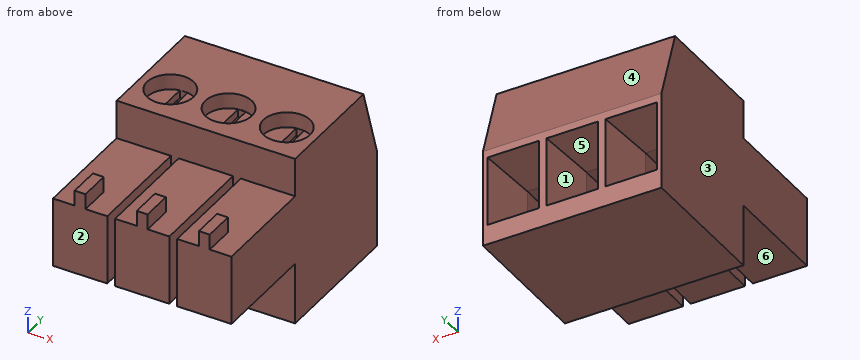
from build123d import *

# Parameters (mm, degrees)
SKETCH1_W                    = 11.5
SKETCH1_H                    = 11
BOSS_EXTRUDE1_DEPTH          = 9
SKETCH2_W                    = 3.5
SKETCH2_H                    = 4.5
BOSS_EXTRUDE2_DEPTH          = 7
SKETCH3_W                    = 3.3
SKETCH3_H                    = 4.5
CUT_EXTRUDE1_DEPTH           = 3
CUT_EXTRUDE1_DRAFT           = -15
CUT_EXTRUDE1_PROFILE_2_DEPTH = 3
CUT_EXTRUDE1_PROFILE_2_DRAFT = -15
CUT_EXTRUDE1_PROFILE_3_DEPTH = 3
CUT_EXTRUDE1_PROFILE_3_DRAFT = -15
SKETCH4_W                    = 1.692304846
SKETCH4_H                    = 2.892304846
CUT_EXTRUDE2_DEPTH           = 3
CUT_EXTRUDE3_DEPTH           = 17
SKETCH6_R                    = 1.5
CUT_EXTRUDE4_DEPTH           = 1
SKETCH7_W                    = 0.5
SKETCH7_H                    = 2.958039891
CUT_EXTRUDE5_DEPTH           = 0.5
SKETCH8_W                    = 0.7
SKETCH8_H                    = 2
BOSS_EXTRUDE3_DEPTH          = 1


with BuildPart() as part:
    # Sketch1 → Boss-Extrude1 (new body)
    with BuildSketch(Plane(origin=(0, 0, 0), x_dir=(1, 0, 0), z_dir=(0, 1, 0))):
        Rectangle(SKETCH1_W, SKETCH1_H)
    extrude(amount=BOSS_EXTRUDE1_DEPTH)

    # Sketch2 → Boss-Extrude2 (add)
    with BuildSketch(Plane.XZ):
        with Locations((-4, 0.75)):
            Rectangle(SKETCH2_W, SKETCH2_H)
        with Locations((4, 0.75)):
            Rectangle(SKETCH2_W, SKETCH2_H)
        with Locations((0, 0.75)):
            Rectangle(SKETCH2_W, SKETCH2_H)
    extrude(amount=BOSS_EXTRUDE2_DEPTH)


with BuildPart() as cut_extrude1_tool:
    # Sketch3 → Cut-Extrude1 (with draft: the straight prism first)
    with BuildSketch(Plane(origin=(0, 9, 0), x_dir=(1, 0, 0), z_dir=(0, 1, 0))):
        with Locations((3.8, 1.95)):
            Rectangle(SKETCH3_W, SKETCH3_H)
    extrude(amount=-CUT_EXTRUDE1_DEPTH)
    # Cut-Extrude1: the draft: its side faces are tilted about the plane it starts from
    cut_extrude1_sides = [cut_extrude1_tool.faces().sort_by_distance(p)[0] for p in [
        (3.8, 7.5, -4.2),
        (2.15, 7.5, -1.95),
        (3.8, 7.5, 0.3),
        (5.45, 7.5, -1.95),
    ]]
    draft(cut_extrude1_sides, Plane(origin=(0, 9, 0), x_dir=(1, 0, 0), z_dir=(0, 1, 0)), CUT_EXTRUDE1_DRAFT)


with BuildPart() as part_1:
    add(part.part)

    # Cut-Extrude1: cut by cut_extrude1_tool
    add(cut_extrude1_tool.part, mode=Mode.SUBTRACT)


with BuildPart() as cut_extrude1_profile_2_tool:
    # Sketch3 → Cut-Extrude1 profile 2 (with draft: the straight prism first)
    with BuildSketch(Plane(origin=(0, 9, 0), x_dir=(1, 0, 0), z_dir=(0, 1, 0))):
        with Locations((-3.8, 1.95)):
            Rectangle(SKETCH3_W, SKETCH3_H)
    extrude(amount=-CUT_EXTRUDE1_PROFILE_2_DEPTH)
    # Cut-Extrude1 profile 2: the draft: its side faces are tilted about the plane it starts from
    cut_extrude1_profile_2_sides = [cut_extrude1_profile_2_tool.faces().sort_by_distance(p)[0] for p in [
        (-3.8, 7.5, -4.2),
        (-5.45, 7.5, -1.95),
        (-3.8, 7.5, 0.3),
        (-2.15, 7.5, -1.95),
    ]]
    draft(cut_extrude1_profile_2_sides, Plane(origin=(0, 9, 0), x_dir=(1, 0, 0), z_dir=(0, 1, 0)), CUT_EXTRUDE1_PROFILE_2_DRAFT)


with BuildPart() as part_2:
    add(part_1.part)

    # Cut-Extrude1 profile 2: cut by cut_extrude1_profile_2_tool
    add(cut_extrude1_profile_2_tool.part, mode=Mode.SUBTRACT)


with BuildPart() as cut_extrude1_profile_3_tool:
    # Sketch3 → Cut-Extrude1 profile 3 (with draft: the straight prism first)
    with BuildSketch(Plane(origin=(0, 9, 0), x_dir=(1, 0, 0), z_dir=(0, 1, 0))):
        with Locations((0, 1.95)):
            Rectangle(SKETCH3_W, SKETCH3_H)
    extrude(amount=-CUT_EXTRUDE1_PROFILE_3_DEPTH)
    # Cut-Extrude1 profile 3: the draft: its side faces are tilted about the plane it starts from
    cut_extrude1_profile_3_sides = [cut_extrude1_profile_3_tool.faces().sort_by_distance(p)[0] for p in [
        (-1.65, 7.5, -1.95),
        (0, 7.5, 0.3),
        (1.65, 7.5, -1.95),
        (0, 7.5, -4.2),
    ]]
    draft(cut_extrude1_profile_3_sides, Plane(origin=(0, 9, 0), x_dir=(1, 0, 0), z_dir=(0, 1, 0)), CUT_EXTRUDE1_PROFILE_3_DRAFT)


with BuildPart() as part_3:
    add(part_2.part)

    # Cut-Extrude1 profile 3: cut by cut_extrude1_profile_3_tool
    add(cut_extrude1_profile_3_tool.part, mode=Mode.SUBTRACT)

    # Sketch4 → Cut-Extrude2 (cut)
    with BuildSketch(Plane(origin=(0, 6, 0), x_dir=(1, 0, 0), z_dir=(0, 1, 0))):
        with Locations((-3.8, 1.95)):
            Rectangle(SKETCH4_W, SKETCH4_H)
        with Locations((3.8, 1.95)):
            Rectangle(SKETCH4_W, SKETCH4_H)
        with Locations((0, 1.95)):
            Rectangle(SKETCH4_W, SKETCH4_H)
    extrude(amount=-CUT_EXTRUDE2_DEPTH, mode=Mode.SUBTRACT)

    # Sketch5 → Cut-Extrude3 (cut)
    with BuildSketch(Plane.ZY.offset(5.75)):
        Polygon((5.5, 9), (0.8, 9), (5.5, 7.5), align=None)
    extrude(amount=-CUT_EXTRUDE3_DEPTH, mode=Mode.SUBTRACT)

    # Sketch6 → Cut-Extrude4 (cut)
    with BuildSketch(Plane.XY.offset(5.5)):
        with Locations((-3.75, 2.487199689)):
            Circle(SKETCH6_R)
        with Locations((0, 2.487199689)):
            Circle(SKETCH6_R)
        with Locations((3.75, 2.487199689)):
            Circle(SKETCH6_R)
    extrude(amount=-CUT_EXTRUDE4_DEPTH, mode=Mode.SUBTRACT)

    # Sketch7 → Cut-Extrude5 (cut)
    with BuildSketch(Plane.XY.offset(4.5)):
        with Locations((-3.75, 2.487199689)):
            Rectangle(SKETCH7_W, SKETCH7_H)
        with Locations((0, 2.487199689)):
            Rectangle(SKETCH7_W, SKETCH7_H)
        with Locations((3.75, 2.487199689)):
            Rectangle(SKETCH7_W, SKETCH7_H)
    extrude(amount=-CUT_EXTRUDE5_DEPTH, mode=Mode.SUBTRACT)

    # Sketch8 → Boss-Extrude3 (add)
    with BuildSketch(Plane.XY.offset(3)):
        with Locations((4, -6)):
            Rectangle(SKETCH8_W, SKETCH8_H)
        with Locations((-4, -6)):
            Rectangle(SKETCH8_W, SKETCH8_H)
        with Locations((0, -6)):
            Rectangle(SKETCH8_W, SKETCH8_H)
    extrude(amount=BOSS_EXTRUDE3_DEPTH)


solid = part_3.part
Geometry: final body of the model. Coordinates: model frame, mm. Face numbers are marked on the shaded views. A direction names the side the tool comes from. Give positions to 0.01 mm unless a question says otherwise; leave off trailing zeros. Order: outer loops, then holes, each group sorted by start corner. A loop starts at its lowest first (then second) coordinate and runs counter-clockwise, first axis right, second up. Notation, with made-up numbers: (31.25, 71) -> (49.25, 71) arc R19 ccw to (49.25, 94) -> close; hole circle Ø10 at (44.25, 14). An arc over 180 degrees is marked (long way). Answer as a JSON object with one key per item and string values.
Q1. Material intervals for probe 1 along X at (y, z) = (-0.25, -0.25); probe 2 along Z at (x, y) = (-4, 4); probe 3 along X at (y, z) = (7, -1.25), sorted ascending.
Entries:
{"probe 1": "x = -5.75 to -2.25, -1.75 to 1.75, 2.25 to 5.75", "probe 2": "z = -5.5 to -3.4, -0.5 to 5.5", "probe 3": "x = -5.75 to -4.91, -2.69 to -1.11, 1.11 to 2.69, 4.91 to 5.75"}
Q2. Section A-A (y = 5.5). Output: boundary loops of the cut face in (x, z).
Entries:
{"outline": "(-5.75, -5.5) -> (5.75, -5.5) -> (5.75, 5.5) -> (-5.75, 5.5) -> close; hole (-4.65, -3.4) -> (-2.95, -3.4) -> (-2.95, -0.5) -> (-4.65, -0.5) -> close; hole (-0.85, -3.4) -> (0.85, -3.4) -> (0.85, -0.5) -> (-0.85, -0.5) -> close; hole (2.95, -3.4) -> (4.65, -3.4) -> (4.65, -0.5) -> (2.95, -0.5) -> close"}
Q3. Draft query along X for the marked faces 1, 2 and 3. Return one class per face: released by +X, released by -X, zero draft, split by the parting line, or undercut.
Entries:
{"face 1": "undercut", "face 2": "zero draft", "face 3": "released by -X"}
Q4. Section D-D (z = 1.75). Output: boundary loops of the cut face in (x, y), plus the area to 3 significant figures.
Entries:
{"outline": "(-5.75, -7) -> (-2.25, -7) -> (-2.25, 0) -> (-1.75, 0) -> (-1.75, -7) -> (1.75, -7) -> (1.75, 0) -> (2.25, 0) -> (2.25, -7) -> (5.75, -7) -> (5.75, 8.7) -> (-5.75, 8.7) -> close", "area": "174 mm^2"}
Q5. Access query for the marked faces 4, 5 and 6. Directions: +Z, -Z, +X, -X, +Y, -Y. A direction counts if a zero-diameter tool reaches every point of the face in a straight line with its end or side. Return the directions, or none.
Entries:
{"face 4": "+Z, +X, -X, +Y", "face 5": "+Y", "face 6": "-Z, +X, -X, -Y"}
Q6. Section B-B (y = -1). Output: boundary loops of the cut face in (x, z), plus the area to 4 significant figures.
Entries:
{"outline": "(-5.75, -1.5) -> (-2.25, -1.5) -> (-2.25, 3) -> (-5.75, 3) -> close; (-1.75, -1.5) -> (1.75, -1.5) -> (1.75, 3) -> (-1.75, 3) -> close; (2.25, -1.5) -> (5.75, -1.5) -> (5.75, 3) -> (2.25, 3) -> close", "area": "47.25 mm^2"}
Q7. First-contact query: pin 1 (0.6 mm diameter, centred on x = 4, z = 4.5, fed in from -Y); pin 2 (1 mm diameter, centred on x = -4.5, y = -3, fed in from +Z); pin 3 (2 mm diameter, centred on x = -0.5, z = 1, fed in from +Y); pin 4 (4 mm diameter, centred on x = 4, y = -4.5, fed in from +Z). Flat tips, straight axial feed; report the tip coordinate or a pass-through.
Entries:
{"pin 1": "stops at y = 0", "pin 2": "stops at z = 3", "pin 3": "stops at y = 9", "pin 4": "stops at z = 4"}
